```python
from build123d import *

# Parameters (mm, degrees)
SKETCH_2_W          = 16
SKETCH_2_H          = 1.5
CUT_EXTRUDE_1_DEPTH = 1


with BuildPart() as part:
    # Эскиз1 → Повернуть1 (revolve)
    with BuildSketch(Plane.XY, mode=Mode.PRIVATE) as revolve_1_sk:
        Polygon((0, 0), (0, 3), (18, 3), (18, 6), (21, 6), (21, 8), (29.5, 8), (29.5, 6), (31, 6), (31, 0), align=None)
    revolve(revolve_1_sk.sketch.rotate(Axis((0, 0, 0), (1, 0, 0)), 90), axis=Axis((0, 0, 0), (1, 0, 0)))

    # Эскиз2 → Вырез-Вытянуть1 (cut)
    with BuildSketch(Plane(origin=(31, 0, 0), x_dir=(0, 0, -1), z_dir=(1, 0, 0))):
        Rectangle(SKETCH_2_W, SKETCH_2_H)
    extrude(amount=-CUT_EXTRUDE_1_DEPTH, mode=Mode.SUBTRACT)


solid = part.part
```
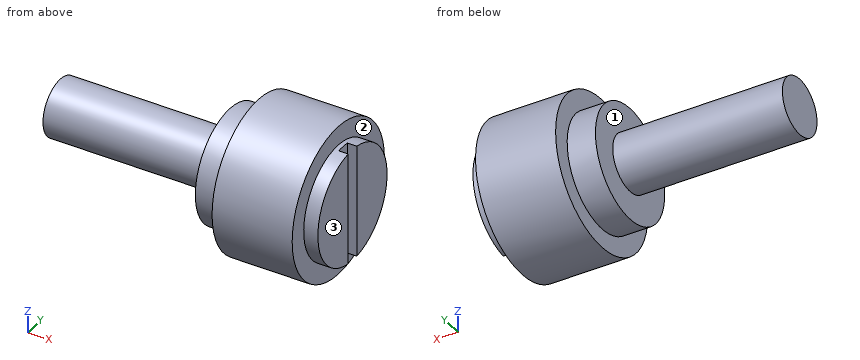
Could you check a few things on this model? Use its own coordinates, in mm. Face numbers are marked on the shaded views. A direction names the side the tool comes from. Give positions to 0.01 mm unless a question says otherwise; leave off trailing zeros. Write each loop counter-clockwise with the first axis right and the second up, starting at its lowest first coordinate (ties: lowest second). Pieces come first, ordered by that corner, then holes. Notation, with made-up numbers: (42, 58.5) - (94, 58.5) arc R30 ccw to (94, 91.5) - close; hole circle Ø11 at (89, -31.75). An arc over 180 degrees is marked (long way). One line per item, written item: value. Start each with the question number.
Item 1: Imagine slicing it at C-C, the plane x = 15.5. List the corners of the cut face in (y, z) for me, and give its area (3 significant figures).
Item 2: Imagine slicing it at D-D, the plane z = 4. List the corners of the cut face in (x, y) for me, and give its area (3 significant figures).
Item 3: Please list where these lines run through material, in increasing order: line 1 (X direction, y = 2.75, z = 1.75); line 2 (X direction, y = -5.5, z = 3.75); line 3 (Y direction, x = 25.5, z = -0.25). Write a range as from..to.
Item 4: I'm going to push flat-ended pins straight in: pin 1 (6 mm diameter, centred on x = 11.5, z = 5, fed in from +Y); pin 2 (1.1 mm diameter, centred on x = 30.5, z = 1.5, fed in from +Y); pin 3 (2 mm diameter, centred on x = 22.5, z = 6.5, fed in from +Y). Where does each tip first touch, or does it pass through?
Item 5: Which directions (+Z, -Z, +X, -X, +Y, -Y) give clear straight access to the entire face, cutting with the end or side of a thin tool? Please do the marked faces 1, 2 and 3.
Item 6: Imagine slicing it at B-B, the plane z = 0. List the corners of the cut face in (x, y) for me, and give its area (4 significant figures).
Item 7: Imagine slicing it at A-A, the plane y = 0. List the corners of the cut face in (x, z) for me.
Geometry says:
1. outline: circle Ø6 at (0, 0)
1. area: 28.3 mm^2
2. outline: (18, -4.47) - (21, -4.47) - (21, -6.93) - (29.5, -6.93) - (29.5, -4.47) - (31, -4.47) - (31, -0.75) - (30, -0.75) - (30, 0.75) - (31, 0.75) - (31, 4.47) - (29.5, 4.47) - (29.5, 6.93) - (21, 6.93) - (21, 4.47) - (18, 4.47) - close
2. area: 157 mm^2
3. line 1: 18..31
3. line 2: 21..29.5
3. line 3: -8..8
4. pin 1: y = 2.24
4. pin 2: y = 5.92
4. pin 3: y = 5.81
5. face 1: -X
5. face 2: +X
5. face 3: +Z, -Z, +X, +Y, -Y
6. outline: (0, -3) - (18, -3) - (18, -6) - (21, -6) - (21, -8) - (29.5, -8) - (29.5, -6) - (31, -6) - (31, -0.75) - (30, -0.75) - (30, 0.75) - (31, 0.75) - (31, 6) - (29.5, 6) - (29.5, 8) - (21, 8) - (21, 6) - (18, 6) - (18, 3) - (0, 3) - close
6. area: 296.5 mm^2
7. outline: (0, -3) - (18, -3) - (18, -6) - (21, -6) - (21, -8) - (29.5, -8) - (29.5, -6) - (30, -6) - (30, 6) - (29.5, 6) - (29.5, 8) - (21, 8) - (21, 6) - (18, 6) - (18, 3) - (0, 3) - close
